```python
from build123d import *

# Parameters (mm, degrees)
F1_DEPTH = 50.8
F2_W     = 61.014819
F2_H     = 64.756295
F2_R     = 9.911554
F3_DEPTH = 25.4


with BuildPart() as f1:
    # F0 (on Front) → F1 (new body)
    with BuildSketch(Plane.XZ):
        Polygon((42.883057, -17.987859), (0, 0), (0, -34.680594), (42.883057, -34.680594), align=None)
    extrude(amount=F1_DEPTH)

    # F2 (on Top) → F3 (cut)
    with BuildSketch(Plane.XY):
        with Locations((21.58543, -24.751295)):
            Rectangle(F2_W, F2_H)
        with Locations((21.873239, -22.592753)):
            Circle(F2_R, mode=Mode.SUBTRACT)
    extrude(amount=-F3_DEPTH, mode=Mode.SUBTRACT)


solid = f1.part
```
The listing builds one solid part. Answer for the finished solid, in the listing's coordinates (mm). A direction names the side the tool comes from. Round coordinates to 2 decimals unless told otherwise and drop trailing zeros. Loops run counter-clockwise (first coordinate to the right, second up) from the corner with the lowest first, then second, coordinate; pieces in that order, holes last.
1) For faces 1 (the face through (21, -50.8, -30)), 2 (the face through (12, -25, -25.4)), determine the directions among +Z, -Z, +X, -X, +Y, -Y from which every point of the face is accessible in a straight line to the end or side of a thin tool.
Outcome:
face 1: +Z, -Z, +X, -X, -Y
face 2: +Z
2) A cutting plane is placed at C-C on z = -24.25. Determine the outline of the cut face in (x, y), plus the area to 3 significant figures.
Outcome:
outline: circle Ø19.82 at (21.87, -22.59)
area: 309 mm2
3) A cutting plane is placed at A-A on y = -30. Determine the outline of the cut face in (x, z), plus the area to 3 significant figures.
Outcome:
outline: (0, -34.68) - (42.88, -34.68) - (42.88, -25.4) - (28.46, -25.4) - (28.46, -11.94) - (15.29, -6.41) - (15.29, -25.4) - (0, -25.4) - close
area: 612 mm2
4) A cutting plane is placed at D-D on x = 38. Determine the outline of the cut face in (y, z).
Outcome:
outline: (-50.8, -34.68) - (0, -34.68) - (0, -25.4) - (-50.8, -25.4) - close
5) Consider line 1 (Z direction, x = 39.5, y = -23.5); line 2 (Y direction, x = 22.5, z = -20); line 3 (X direction, y = -30, z = -18.5). Determine where each line is inside the solid, lowest interval first.
Outcome:
line 1: z = -34.68 to -25.4
line 2: y = -32.48 to -12.7
line 3: x = 15.29 to 28.46
6) Given P1, Ø5, axis at x = 27, z = -21, coming from the -Y side; P2, Ø3, axis at y = -30.5, z = -16, coming from the -X side; P3, Ø2, axis at x = 20.5, z = -11, coming from the +Y side, each flat-ended and moving along its own axis, determine where each tip first touches the part or whether it passes through.
Outcome:
P1: stops at y = -32.15
P2: stops at x = 14.31
P3: stops at y = -12.69
7) A cutting plane is placed at B-B on x = 16.5. Determine the outline of the cut face in (y, z), plus the area to 3 significant figures.
Outcome:
outline: (-50.8, -34.68) - (0, -34.68) - (0, -25.4) - (-14.26, -25.4) - (-14.26, -6.92) - (-30.92, -6.92) - (-30.92, -25.4) - (-50.8, -25.4) - close
area: 779 mm2
